from build123d import *

# Parameters (mm, degrees)
F0_W     = 71.607996
F0_H     = 68.552719
F1_DEPTH = 50.8
F4_DEPTH = 25.4


with BuildPart() as f1:
    # F0 (on Front) → F1 (new body)
    with BuildSketch(Plane.XZ):
        with Locations((-3.246227, 5.155774)):
            Rectangle(F0_W, F0_H)
    extrude(amount=F1_DEPTH)

    # F3 (on face) → F4 (join)
    with BuildSketch(Plane.XZ.offset(50.8)):
        Polygon((-39.050225, -5.824117), (-38.668316, -28.92963), (-17.281396, -28.92963), (-17.281396, -5.824117), align=None)
    extrude(amount=F4_DEPTH)


solid = f1.part
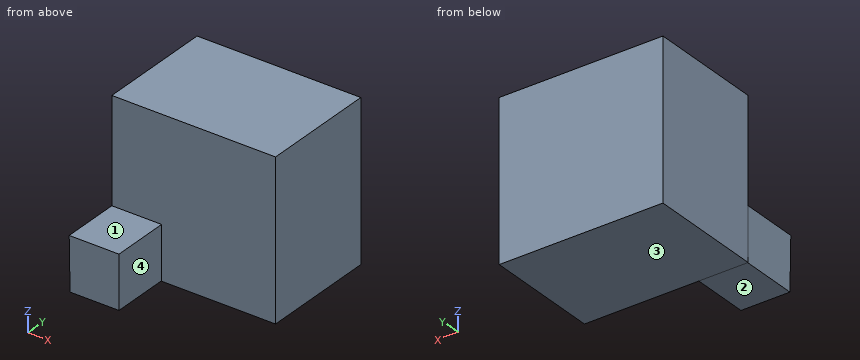
Here's how the part is built. I have some questions about the finished solid (model axes, mm). Face numbers are marked on the shaded views. A direction names the side the tool comes from. Give positions to 0.01 mm unless a question says otherwise; leave off trailing zeros. Loops run counter-clockwise (first coordinate to the right, second up) from the corner with the lowest first, then second, coordinate; pieces in that order, holes last. Notation, with made-up numbers: (19.25, -9.75) -> (69.25, -9.75) arc R13 ccw to (69.25, 11.25) -> close; hole circle Ø3 at (0.5, 45). An arc over 180 degrees is marked (long way). Answer as a JSON object with one key per item and string values. Group by question number.
Item 1: I need wall thicknesses on L1, parallel to Y at x = -9, z = -3.5; L2, parallel to Z at x = -22, y = -72; L3, parallel to X at y = -51.5, z = -26. Which ranges of each line are inside material? Lowest first, please.
Item 2: Will these pins go through, and if not, where does the flat tip stop? pin 1 (11.5 mm diameter, centred on y = -67, z = -16.5, fed in from +X); pin 2 (17.5 mm diameter, centred on x = -31.5, y = -62.5, fed in from +Z); pin 3 (17 mm diameter, centred on x = -26.5, y = -65, fed in from -Z).
Item 3: Imagine slicing it at D-D on z = 20. Write out the boundary of the cut face in (x, y).
Item 4: Imagine slicing it at A-A on x = -29. Write out the boundary of the cut face in (y, z), then the cut area to 3 significant figures.
Item 5: Imagine slicing it at C-C on y = -71. Write out the boundary of the cut face in (x, z).
Item 6: On a 3-axis mill with a long thin cutter (end or side, diameter ignored), from which of +Z, -Z, +X, -X, +Y, -Y can I reach the whole of each face in a straight line? I mean the marked faces 1, 2, 3 and 4. Say none if no direction works.
Item 7: Imagine slicing it at B-B on z = -12. Write out the boundary of the cut face in (x, y).
Answer list:
{
 "1": {"L1": "y = -50.8 to 0", "L2": "z = -28.93 to -5.82", "L3": "x = -38.72 to -17.28"},
 "2": {"pin 1": "stops at x = -17.28", "pin 2": "stops at z = -5.82", "pin 3": "stops at z = -28.93"},
 "3": {"outline": "(-39.05, -50.8) -> (32.56, -50.8) -> (32.56, 0) -> (-39.05, 0) -> close"},
 "4": {"outline": "(-76.2, -28.93) -> (-50.8, -28.93) -> (-50.8, -29.12) -> (0, -29.12) -> (0, 39.43) -> (-50.8, 39.43) -> (-50.8, -5.82) -> (-76.2, -5.82) -> close", "area": "4,070 mm2"},
 "5": {"outline": "(-39.05, -5.82) -> (-38.67, -28.93) -> (-17.28, -28.93) -> (-17.28, -5.82) -> close"},
 "6": {"face 1": "+Z, +X, -X, -Y", "face 2": "-Z, +X, -X, -Y", "face 3": "-Z, +X, -X, +Y, -Y", "face 4": "+Z, -Z, +X, -Y"},
 "7": {"outline": "(-39.05, -50.8) -> (-38.95, -50.8) -> (-38.95, -76.2) -> (-17.28, -76.2) -> (-17.28, -50.8) -> (32.56, -50.8) -> (32.56, 0) -> (-39.05, 0) -> close"}
}
